from build123d import *

# Parameters (mm, degrees)
SKETCH_1_W                  = 84
SKETCH_1_H                  = 80
SKETCH_1_R                  = 13.9
EXTRUDE_1_DEPTH             = 5
EXTRUDE_2_DEPTH             = 22
CUT_EXTRUDE_3_REACH         = 79
HOLE_START                  = -42
HOLE_WIZARD_2_OUTLINE_R     = 1.7
HOLE_WIZARD_2_DEPTH         = 11
HOLE_WIZARD_2_2_OUTLINE_R   = 3
HOLE_WIZARD_2_2_OUTLINE_R_2 = 1.7
HOLE_WIZARD_2_2_DEPTH       = 3.4
HOLE_WIZARD_M4_2_D          = 3.3
SKETCH_14_R                 = 38
SKETCH_14_R_2               = 33
CUT_EXTRUDE_4_DEPTH         = 4
HOLE_WIZARD_3_D             = 3.2
HOLE_WIZARD_3_CBORE_D       = 6
HOLE_WIZARD_3_CBORE_DEPTH   = 3.4
CHAMFER_1_SIZE              = 23
SKETCH_17_R                 = 14.5
CUT_EXTRUDE_5_DEPTH         = 6
SKETCH_18_R                 = 33
CUT_EXTRUDE_6_DEPTH         = 2


# Read off the part's stored shape, not the designer's step: 打孔尺寸(%根据)内六角圆柱头螺钉的类型2
with BuildPart() as part:
    # 草图1 → 凸台-拉伸1 (new, symmetric)
    with BuildSketch(Plane.XY):
        Rectangle(SKETCH_1_W, SKETCH_1_H)
        Circle(SKETCH_1_R, mode=Mode.SUBTRACT)
    extrude(amount=EXTRUDE_1_DEPTH, both=True)

    # 草图6 → 凸台-拉伸2 (add)
    with BuildSketch(Plane.ZY.offset(42)):
        Polygon((-5, -14.766158372), (-5, -40), (-30, -40), (-33.816179908, -20.367456331), align=None)
    extrude_2 = extrude(amount=-EXTRUDE_2_DEPTH)

    # 切除-拉伸3: up to this plane
    cut_extrude_3_end = Plane(origin=(-42, -40, 5), z_dir=(0, 1, 0))
    # 草图7 → 切除-拉伸3 (cut, up to the surface)
    with BuildSketch(Plane(origin=(0, -13.292034521, 2.583709779), x_dir=(1, 0, 0), z_dir=(0, 0.9816271834476648, -0.19080899537654153)), mode=Mode.PRIVATE) as cut_extrude_3_sk1:
        with BuildLine():
            Line((-31, 37.081175318), (-29, 37.081175318))
            Line((-29, 37.081175318), (-29, 29.662905695))
            ThreePointArc((-29, 29.662905695), (-30, 13.725651762), (-31, 29.662905695))
            Line((-31, 29.662905695), (-31, 37.081175318))
        make_face()
    cut_extrude_3_tool1 = split(extrude(cut_extrude_3_sk1.sketch, amount=-CUT_EXTRUDE_3_REACH, mode=Mode.PRIVATE), bisect_by=cut_extrude_3_end, keep=Keep.BOTH, mode=Mode.PRIVATE)
    cut_extrude_3 = cut_extrude_3_tool1.solids().sort_by_distance((-30, -17.589666, -19.525688))[0]
    add(cut_extrude_3, mode=Mode.SUBTRACT)

    # 打孔尺寸(%根据)内六角圆柱头螺钉的类型2 outline → 打孔尺寸(%根据)内六角圆柱头螺钉的类型2 (cut)
    with BuildSketch(Plane.YZ.offset(HOLE_START)):
        with Locations((-35.310255285, -26.836727248)):
            Circle(HOLE_WIZARD_2_OUTLINE_R)
        with Locations((-24.512356267, -28.935626197)):
            Circle(HOLE_WIZARD_2_OUTLINE_R)
    hole_wizard_2 = extrude(amount=HOLE_WIZARD_2_DEPTH, mode=Mode.SUBTRACT)

    # Hole Wizard 2 2 outline → Hole Wizard 2 2 (cut)
    # profile 1 of 2: a face of its own
    with BuildSketch(Plane.YZ.offset(HOLE_START)):
        with Locations((-35.310255285, -26.836727248)):
            Circle(HOLE_WIZARD_2_2_OUTLINE_R)
        with Locations((-35.310255285, -26.836727248)):
            Circle(HOLE_WIZARD_2_2_OUTLINE_R_2, mode=Mode.SUBTRACT)
    # profile 2 of 2: a face of its own
    with BuildSketch(Plane.YZ.offset(HOLE_START)):
        with Locations((-24.512356267, -28.935626197)):
            Circle(HOLE_WIZARD_2_2_OUTLINE_R)
        with Locations((-24.512356267, -28.935626197)):
            Circle(HOLE_WIZARD_2_2_OUTLINE_R_2, mode=Mode.SUBTRACT)
    hole_wizard_2_2 = extrude(amount=HOLE_WIZARD_2_2_DEPTH, mode=Mode.SUBTRACT)

    # M4 螺纹孔2 (through all)
    with Locations(Plane(origin=(-20, 0, 0), x_dir=(0, 0, -1), z_dir=(1, 0, 0))):
        with Locations((28.935626197, -24.512356267), (26.836727248, -35.310255285)):
            hole_wizard_m4_2 = Hole(HOLE_WIZARD_M4_2_D / 2)

    # 草图14 → 切除-拉伸4 (cut)
    with BuildSketch(Plane.XY.offset(5)):
        Circle(SKETCH_14_R)
        Circle(SKETCH_14_R_2, mode=Mode.SUBTRACT)
    extrude(amount=-CUT_EXTRUDE_4_DEPTH, mode=Mode.SUBTRACT)

    # 镜向1: 凸台-拉伸2, 切除-拉伸3, 打孔尺寸(%根据)内六角圆柱头螺钉的类型2, Hole Wizard 2 2, M4 螺纹孔2 across plane
    add(extrude_2.mirror(Plane(origin=(0, 0, 0), x_dir=(0, 0, 1), z_dir=(1, 0, 0))))
    add(cut_extrude_3.mirror(Plane(origin=(0, 0, 0), x_dir=(0, 0, 1), z_dir=(1, 0, 0))), mode=Mode.SUBTRACT)
    add(hole_wizard_2.mirror(Plane(origin=(0, 0, 0), x_dir=(0, 0, 1), z_dir=(1, 0, 0))), mode=Mode.SUBTRACT)
    add(hole_wizard_2_2.mirror(Plane(origin=(0, 0, 0), x_dir=(0, 0, 1), z_dir=(1, 0, 0))), mode=Mode.SUBTRACT)
    add(hole_wizard_m4_2.mirror(Plane(origin=(0, 0, 0), x_dir=(0, 0, 1), z_dir=(1, 0, 0))), mode=Mode.SUBTRACT)

    # 打孔尺寸(%根据)内六角圆柱头螺钉的类型3 (through all)
    with Locations(Plane(origin=(0, 0, -5), x_dir=(-1, 0, 0), z_dir=(0, 0, -1))):
        with Locations((0, 35.5), (35.5, 0), (0, -35.5), (-35.5, 0)):
            CounterBoreHole(HOLE_WIZARD_3_D / 2, HOLE_WIZARD_3_CBORE_D / 2, HOLE_WIZARD_3_CBORE_DEPTH)

    # 倒角1
    chamfer_1_edges = [part.edges().sort_by_distance(p)[0] for p in [
        (42, 40, 0),
        (-42, 40, 0),
    ]]
    chamfer(chamfer_1_edges, length=CHAMFER_1_SIZE)

    # 草图17 → 切除-拉伸5 (cut)
    with BuildSketch(Plane.XY.offset(5)):
        Circle(SKETCH_17_R)
    extrude(amount=-CUT_EXTRUDE_5_DEPTH, mode=Mode.SUBTRACT)

    # 草图18 → 切除-拉伸6 (cut)
    with BuildSketch(Plane.XY.offset(5)):
        Circle(SKETCH_18_R)
    extrude(amount=-CUT_EXTRUDE_6_DEPTH, mode=Mode.SUBTRACT)


solid = part.part
Work out the finished part from the listing and answer in its coordinate system (mm). A direction names the side the tool comes from. Give positions to 0.01 mm unless a question says otherwise; leave off trailing zeros. Write each loop counter-clockwise with the first axis right and the second up, starting at its lowest first coordinate (ties: lowest second). Pieces come first, ordered by that corner, then holes.
Q1. The part is cut by section D-D on x = 35.5. Give the vertices of the cut face in (y, z).
Answer:
outline: (-40, -30) - (-20.37, -33.82) - (-18.55, -24.45) - (-40, -20.28) - close; (-40, -8.44) - (-16.33, -13.04) - (-14.77, -5) - (-3, -5) - (-3, -1.6) - (-1.6, -1.6) - (-1.6, 1) - (-13.56, 1) - (-13.56, 5) - (-40, 5) - close; (1.6, -1.6) - (3, -1.6) - (3, -5) - (23.5, -5) - (23.5, 5) - (13.56, 5) - (13.56, 1) - (1.6, 1) - close; hole circle Ø3.4 at (-35.31, -26.84); hole circle Ø3.4 at (-24.51, -28.94)
Q2. The part is cut by section C-C on x = -26. Give the vertices of the cut face in (y, z), and give its area (3 significant figures).
Answer:
outline: (-40, -30) - (-20.37, -33.82) - (-18.76, -25.54) - (-40, -21.41) - close; (-40, -7.3) - (-16.12, -11.94) - (-14.77, -5) - (33, -5) - (33, 5) - (27.71, 5) - (27.71, 1) - (20.32, 1) - (20.32, 3) - (-20.32, 3) - (-20.32, 1) - (-27.71, 1) - (-27.71, 5) - (-40, 5) - close; hole circle Ø3.3 at (-35.31, -26.84); hole circle Ø3.3 at (-24.51, -28.94)
area: 863 mm2
Q3. Given pin 1 (3 mm diameter, centred on y = -35.5, z = -25.5, fed in from +X); pin 2 (4 mm diameter, centred on x = 0, y = -35.5, fed in from +Z); pin 3 (3 mm diameter, centred on y = -24, z = -29, fed in from -X), each flat-ended and moving along its own axis, determine where each tip first touches the part or whether it passes through.
Answer:
pin 1: stops at x = 38.6
pin 2: stops at z = 1
pin 3: stops at x = -38.6
Q4. For a pull along Y with two mould halves and no side action, classify faces 1 (the face through (33.9, 0.07, -0.28)), 2 (the face through (-31, -30, -28)), 3 (the face through (0, 40, 0)) as released by +Y, released by -Y, zero draft, split by the parting line, or undercut.
Answer:
face 1: undercut
face 2: zero draft
face 3: released by +Y
Q5. A tool of negligible diameter and unlimited length cuts with its end or side. For faces 4 (the face through (40.324, -32.449, -25.936)), 5 (the face through (-1, -37, -1.6)), 6 (the face through (-11.44, 31.14, 1)), 7 (the face through (-38.6, -33, -27)), from which of +Z, -Z, +X, -X, +Y, -Y can it reach the whole face along a straight path? Write none if from no direction.
Answer:
face 4: +X
face 5: -Z
face 6: +Z
face 7: -X
Q6. The part is cut by section A-A on x = -5.5. Give the vertices of the cut face in (y, z), and give its area (3 significant figures).
Answer:
outline: (-40, -5) - (-12.77, -5) - (-12.77, -1) - (-13.42, -1) - (-13.42, 3) - (-32.54, 3) - (-32.54, 1) - (-37.6, 1) - (-37.6, 5) - (-40, 5) - close; (12.77, -5) - (40, -5) - (40, 5) - (37.6, 5) - (37.6, 1) - (32.54, 1) - (32.54, 3) - (13.42, 3) - (13.42, -1) - (12.77, -1) - close
area: 420 mm2
Q7. Straight lines are drawn through the part: L1, parallel to Y at x = 0, z = 0; L2, parallel to X at y = -34, z = -31; L3, parallel to Y at x = 0, z = -2.6. For each, find the intervals that lie inside material, in ascending order.
Answer:
L1: y = -40 to -37.1, -33.9 to -14.5, 14.5 to 33.9, 37.1 to 40
L2: x = -42 to -31, -29 to -20, 20 to 29, 31 to 42
L3: y = -40 to -38.5, -32.5 to -13.9, 13.9 to 32.5, 38.5 to 40
Q8. The part is cut by section B-B on y = 35.5. Give the vertices of the cut face in (x, z), and give its area (3 significant figures).
Answer:
outline: (-23.5, -5) - (-3, -5) - (-3, -1.6) - (-1.6, -1.6) - (-1.6, 1) - (-13.56, 1) - (-13.56, 5) - (-23.5, 5) - close; (1.6, -1.6) - (3, -1.6) - (3, -5) - (23.5, -5) - (23.5, 5) - (13.56, 5) - (13.56, 1) - (1.6, 1) - close
area: 333 mm2
